from build123d import *

# Parameters (mm, degrees)
F1_DEPTH = 15
F2_R     = 1


with BuildPart() as f1:
    # F0 (on Top) → F1 (new body)
    with BuildSketch(Plane.XY):
        with BuildLine():
            Line((-70, -35), (-70, 0))
            Line((-70, 0), (65, 0))
            Line((65, 0), (65, -9))
            Line((65, -9), (155.40206, -9))
            Line((155.40206, -9), (155.40206, 0))
            Line((155.40206, 0), (77.26491, 34.468791))
            ThreePointArc((77.26491, 34.468791), (85.791563, 9.361335), (60.050126, 3))
            Line((60.050126, 3), (-73, 3))
            Line((-73, 3), (-73, -38))
            Line((-73, -38), (-30, -38))
            Line((-30, -38), (-30, -35))
            Line((-30, -35), (-70, -35))
        make_face()
        with BuildLine():
            ThreePointArc((60.050126, 3), (85.791563, 9.361335), (77.26491, 34.468791))
            ThreePointArc((77.26491, 34.468791), (73.71226, 35.613038), (70, 36))
            Line((70, 36), (70, 33))
            ThreePointArc((70, 33), (85, 18), (70, 3))
            Line((70, 3), (60.050126, 3))
        make_face()
    extrude(amount=F1_DEPTH)

    # F2
    f2_edges = [f1.edges().sort_by_distance(p)[0] for p in [
        (65, -9, 7.5),
        (155.40206, -9, 7.5),
        (155.40206, 0, 7.5),
        (-30, -35, 7.5),
    ]]
    fillet(f2_edges, radius=F2_R)


solid = f1.part
CAD build for the part. Positions are in the model's coordinates, mm. A direction names the side the tool comes from. Coordinates: 2 decimals unless noted, no trailing zeros. Order: outer loops, then holes, each group sorted by start corner. A loop starts at its lowest first (then second) coordinate and runs counter-clockwise, first axis right, second up.
Item 1: Drill centre lines: L1, parallel to Y at x = -55, z = 10.25; L2, parallel to X at y = -31, z = 9.75; L3, parallel to Y at x = 56, z = 11.5. Where is each one in solid material? Low to high.
Check sheet entries:
L1: y = -38 to -35, 0 to 3
L2: x = -73 to -70
L3: y = 0 to 3
Item 2: Two-plate mould, pull along X, no slides. Class faces 5 (the face through (110, -9, 7)), 6 (the face through (-70, -18, 7)), 7 (the face through (-73, -17, 7)): +X half, -X half, draft (parallel to the pull), parting line (faces both ways), or undercut.
Check sheet entries:
face 5: draft
face 6: undercut
face 7: -X half
Item 3: Band-saw the part on D-D on y = -15. List the corners of the cut face in (x, z).
Check sheet entries:
outline: (-73, 0) - (-70, 0) - (-70, 15) - (-73, 15) - close
Item 4: Pin check, flat tips, straight feed: pin 1 Ø5 at (x, z) = (44.5, 3) entering from +Y; pin 2 Ø6 at (x, y) = (80, -5) entering from -Z; pin 3 Ø0.9 at (y, z) = (34.5, 10) entering from -X; pin 4 Ø4.5 at (y, z) = (-22.5, 7) entering from +X. Stop position of each tip, or through.
Check sheet entries:
pin 1: stops at y = 3
pin 2: stops at z = 0
pin 3: stops at x = 70
pin 4: stops at x = -70
Item 5: 3-axis set-ups, long thin cutter, end or side, ignore diameter. For faces 1 (the face through (65, -4, 7)), 2 (the face through (-50, -35, 7)), 3 (the face through (0, 3, 7)), 4 (the face through (-3, 0, 7)): which of +Z, -Z, +X, -X, +Y, -Y reach the whole face in a straight line?
Check sheet entries:
face 1: +Z, -Z, -Y
face 2: +Z, -Z, +X
face 3: +Z, -Z, -X, +Y
face 4: +Z, -Z
Item 6: Band-saw the part on B-B on z = 4. List the corners of the cut face in (x, y), plus the area to 3 significant figures.
Check sheet entries:
outline: (-73, -38) - (-30, -38) - (-30, -36) arc R1 ccw to (-31, -35) - (-70, -35) - (-70, 0) - (65, 0) - (65, -8) arc R1 ccw to (66, -9) - (154.4, -9) arc R1 ccw to (155.4, -8) - (155.4, -0.65) arc R1 ccw to (154.81, 0.26) - (77.26, 34.47) arc R18 ccw to (70, 36) - (70, 33) arc R15 cw to (70, 3) - (-73, 3) - close
area: 2,730 mm2
Item 7: Band-saw the part on A-A on x = -56. List the corners of the cut face in (y, z), plus the area to 3 significant figures.
Check sheet entries:
outline: (-38, 0) - (-35, 0) - (-35, 15) - (-38, 15) - close; (0, 0) - (3, 0) - (3, 15) - (0, 15) - close
area: 90.0 mm2
Item 8: Band-saw the part on C-C on x = 36. List the corners of the cut face in (y, z).
Check sheet entries:
outline: (0, 0) - (3, 0) - (3, 15) - (0, 15) - close
